Verification items for the finished model (mm, model axes). A direction names the side the tool comes from. Round coordinates to 2 decimals unless told otherwise and drop trailing zeros. Write each loop counter-clockwise with the first axis right and the second up, starting at its lowest first coordinate (ties: lowest second). Pieces come first, ordered by that corner, then holes.
from build123d import *

# Parameters (mm, degrees)
T_LE_DE_BASE_PLI_E1_DEPTH             = 20.5
ESQUISSE8_W                           = 24
ESQUISSE8_H                           = 2
BOSS_EXTRU_1_DEPTH                    = 8.5
T_LE_PLI_E_SUR_AR_TE1_STRIP_W         = 10
T_LE_PLI_E_SUR_AR_TE1_STRIP_H         = 2
T_LE_PLI_E_SUR_AR_TE1_STRIP_CUT_DEPTH = 8.5
T_LE_PLI_E_SUR_AR_TE1_DEPTH           = 8.5
ESQUISSE12_W                          = 1.5
ESQUISSE12_H                          = 12
ENL_V_MAT_EXTRU_1_DEPTH               = 8.5
DIAM_TRE_DU_PER_AGE_4_0_4_1_D         = 4
DIAM_TRE_DU_PER_AGE_8_0_8_1_D         = 8
DIAM_TRE_DU_PER_AGE_2_5_2_5_1_D       = 2.5
R_P_TITION_CIRCULAIRE1_COUNT          = 8
DIAM_TRE_DU_PER_AGE_4_0_4_2_D         = 4
DIAM_TRE_DU_PER_AGE_2_5_2_5_2_D       = 2.5
CONG_1_R                              = 4
DIAM_TRE_DU_PER_AGE_8_0_8_2_D         = 8
DIAM_TRE_DU_PER_AGE_2_5_2_5_3_D       = 2.5
R_P_TITION_CIRCULAIRE2_COUNT          = 4
CUT_EXTRUDE1_DEPTH                    = 54.200093985
CUT_EXTRUDE1_DEPTH_BACK               = 54.200093985
SKETCH1_R                             = 1.25


# Sheet-metal steps are written as plain solids
with BuildPart() as part:
    # Esquisse1 → Tôle de base pliée1 (new body)
    with BuildSketch(Plane(origin=(0, 0, 0), x_dir=(0, 0, -1), z_dir=(1, 0, 0))):
        with BuildLine():
            Line((0, 27), (0, 3))
            ThreePointArc((0, 3), (-0.878679656, 0.878679656), (-3, 0))
            Line((-3, 0), (-37.5, 0))
            Line((-37.5, 0), (-37.5, 2))
            Line((-37.5, 2), (-3, 2))
            ThreePointArc((-3, 2), (-2.292893219, 2.292893219), (-2, 3))
            Line((-2, 3), (-2, 27))
            Line((-2, 27), (0, 27))
        make_face()
    extrude(amount=T_LE_DE_BASE_PLI_E1_DEPTH)

    # Esquisse8 → Boss.-Extru.1 (add)
    with BuildSketch(Plane(origin=(20.5, 0, 0), x_dir=(0, 0, -1), z_dir=(1, 0, 0))):
        with Locations((-19, 1)):
            Rectangle(ESQUISSE8_W, ESQUISSE8_H)
    extrude(amount=BOSS_EXTRU_1_DEPTH)

    # Tôle pliée sur arête1 strip (across the edge) → Tôle pliée sur arête1 strip cut (cut)
    with BuildSketch(Plane(origin=(20.5, 2, 31), x_dir=(0, 0, -1), z_dir=(1, 0, 0))):
        with Locations((-4, -1)):
            Rectangle(T_LE_PLI_E_SUR_AR_TE1_STRIP_W, T_LE_PLI_E_SUR_AR_TE1_STRIP_H)
    extrude(amount=T_LE_PLI_E_SUR_AR_TE1_STRIP_CUT_DEPTH, mode=Mode.SUBTRACT)

    # Tôle pliée sur arête1 section (across the edge) → Tôle pliée sur arête1 (add)
    with BuildSketch(Plane(origin=(20.5, 2, 31), x_dir=(0, 0, -1), z_dir=(1, 0, 0))):
        with BuildLine():
            Line((-2, 1), (-2, 25))
            Line((-2, 25), (0, 25))
            Line((0, 25), (0, 1))
            ThreePointArc((0, 1), (0.292893219, 0.292893219), (1, 0))
            Line((1, 0), (1, -2))
            ThreePointArc((1, -2), (-1.121320344, -1.121320344), (-2, 1))
        make_face()
    extrude(amount=T_LE_PLI_E_SUR_AR_TE1_DEPTH)

    # Esquisse12 → Enlèv. mat.-Extru.1 (cut)
    with BuildSketch(Plane(origin=(0, 2, 0), x_dir=(1, 0, 0), z_dir=(0, 1, 0))):
        with Locations((19.75, -31.5)):
            Rectangle(ESQUISSE12_W, ESQUISSE12_H)
    extrude(amount=-ENL_V_MAT_EXTRU_1_DEPTH, mode=Mode.SUBTRACT)

    # Diamètre du perçage Ø4.0 (4)1 (through all)
    with Locations(Plane(origin=(0, 2, 0), x_dir=(1, 0, 0), z_dir=(0, 1, 0))):
        with Locations((24.25, -12.13), (24.25, -22.13)):
            Hole(DIAM_TRE_DU_PER_AGE_4_0_4_1_D / 2)

    # Diamètre du perçage Ø8.0 (8)1 (through all)
    with Locations(Plane(origin=(0, 2, 0), x_dir=(1, 0, 0), z_dir=(0, 1, 0))):
        with Locations((9.75, -25.5)):
            Hole(DIAM_TRE_DU_PER_AGE_8_0_8_1_D / 2)

    # Diamètre du perçage Ø2.5 (2.5)1 (through all)
    with Locations(Plane(origin=(0, 2, 0), x_dir=(1, 0, 0), z_dir=(0, 1, 0))):
        with Locations((9.75, -18.5)):
            diam_tre_du_per_age_2_5_2_5_1 = Hole(DIAM_TRE_DU_PER_AGE_2_5_2_5_1_D / 2)

    # Répétition circulaire1: Diamètre du perçage Ø2.5 (2.5)1 ×8 about axis, 3 skipped
    r_p_tition_circulaire1_axis = Axis((9.75, 2, 25.5), (0, 1, 0))
    add([diam_tre_du_per_age_2_5_2_5_1.rotate(r_p_tition_circulaire1_axis, i * 360 / R_P_TITION_CIRCULAIRE1_COUNT) for i in range(1, R_P_TITION_CIRCULAIRE1_COUNT) if i not in (1, 3, 6)], mode=Mode.SUBTRACT)

    # Diamètre du perçage Ø4.0 (4)2 (through all)
    with Locations(Plane.XY.offset(33)):
        with Locations((24.25, 19.87), (24.25, 9.87)):
            Hole(DIAM_TRE_DU_PER_AGE_4_0_4_2_D / 2)

    # Diamètre du perçage Ø2.5 (2.5)2 (through all)
    with Locations(Plane.XY.offset(2)):
        with Locations((10, 14.87)):
            Hole(DIAM_TRE_DU_PER_AGE_2_5_2_5_2_D / 2)

    # Congé1
    cong_1_edges = [part.edges().sort_by_distance(p)[0] for p in [
        (20.5, 27, 1),
        (29, 1, 7),
        (29, 27, 32),
        (19, 1, 37.5),
    ]]
    fillet(cong_1_edges, radius=CONG_1_R)

    # Symétrie1: part across plane


with BuildPart() as part_1:
    add(part.part)
    add(part.part.mirror(Plane(origin=(0, 3, 3), x_dir=(0, 0, 1), z_dir=(1, 0, 0))))

    # Diamètre du perçage Ø8.0 (8)2 (through all)
    with Locations(Plane(origin=(0, 2, 0), x_dir=(1, 0, 0), z_dir=(0, 1, 0))):
        with Locations((0, -12.13)):
            Hole(DIAM_TRE_DU_PER_AGE_8_0_8_2_D / 2)

    # Diamètre du perçage Ø2.5 (2.5)3 (through all)
    with Locations(Plane(origin=(0, 2, 0), x_dir=(1, 0, 0), z_dir=(0, 1, 0))):
        with Locations((0, -5.13)):
            diam_tre_du_per_age_2_5_2_5_3 = Hole(DIAM_TRE_DU_PER_AGE_2_5_2_5_3_D / 2)

    # Répétition circulaire2: Diamètre du perçage Ø2.5 (2.5)3 ×4 about axis
    r_p_tition_circulaire2_axis = Axis((0, 0, 12.13), (0, 1, 0))
    for i in range(1, R_P_TITION_CIRCULAIRE2_COUNT):
        add(diam_tre_du_per_age_2_5_2_5_3.rotate(r_p_tition_circulaire2_axis, i * 360 / R_P_TITION_CIRCULAIRE2_COUNT), mode=Mode.SUBTRACT)

    # Sketch1 → Cut-Extrude1 (cut, two sides: drawn at the far end of the back side and taken through both)
    with BuildSketch(Plane.XY.offset(2).offset(-CUT_EXTRUDE1_DEPTH_BACK)):
        with Locations((-10, 21.87)):
            Circle(SKETCH1_R)
        with Locations((-3, 14.87)):
            Circle(SKETCH1_R)
        with Locations((-10, 7.87)):
            Circle(SKETCH1_R)
        with Locations((-17, 14.87)):
            Circle(SKETCH1_R)
        with Locations(Location((3, 14.87, 0), (0, 0, 90))):
            Circle(SKETCH1_R)
        with Locations(Location((10, 7.87, 0), (0, 0, 90))):
            Circle(SKETCH1_R)
        with Locations(Location((17, 14.87, 0), (0, 0, 90))):
            Circle(SKETCH1_R)
        with Locations(Location((10, 21.87, 0), (0, 0, 90))):
            Circle(SKETCH1_R)
    extrude(amount=CUT_EXTRUDE1_DEPTH + CUT_EXTRUDE1_DEPTH_BACK, mode=Mode.SUBTRACT)


solid = part_1.part
Q1. Depth check by flat-ended pin: P1, Ø2, axis at x = 2.75, z = 25.5, coming from the +Y side; P2, Ø4, axis at y = 14, z = 30.5, coming from the -X side; P3, Ø12, axis at x = -7.5, z = 30.5, coming from the +Y side; P4, Ø8, axis at y = 11, z = 5.5, coming from the -X side. Enter the tip coordinate at first touch or a pass-through.
Recorded:
P1: passes through
P2: stops at x = -29
P3: stops at y = 2
P4: stops at x = -20.5
Q2. Material ranges on line 1 along Z through (x, y) = (-9.75, 1); line 2 along Y through (x, z) = (-24.25, 32.5); line 3 along X through (y, z) = (0.8, 5.13), recorded low to high.
Recorded:
line 1: z = 0.76 to 17.25, 19.75 to 21.5, 29.5 to 31.25, 33.75 to 37.5
line 2: y = 1.34 to 7.87, 11.87 to 17.87, 21.87 to 27
line 3: x = -20.5 to -1.25, 1.25 to 20.5
Q3. Sectioned sample at A-A (y = 5.75). Enter the section's corners in (x, z).
Recorded:
outline: (-29, 31) - (-20.5, 31) - (-20.5, 33) - (-29, 33) - close; (-20.5, 0) - (20.5, 0) - (20.5, 2) - (-20.5, 2) - close; (20.5, 31) - (29, 31) - (29, 33) - (20.5, 33) - close
Q4. Sectioned sample at B-B (x = -24.25). Enter the section's corners in (y, z), plus the area to 3 significant figures.
Recorded:
outline: (0, 7) - (2, 7) - (2, 10.13) - (0, 10.13) - close; (0, 14.13) - (2, 14.13) - (2, 20.13) - (0, 20.13) - close; (0, 24.13) - (2, 24.13) - (2, 30) arc R1 cw to (3, 31) - (7.87, 31) - (7.87, 33) - (3, 33) arc R3 ccw to (0, 30) - close; (11.87, 31) - (17.87, 31) - (17.87, 33) - (11.87, 33) - close; (21.87, 31) - (27, 31) - (27, 33) - (21.87, 33) - close
area: 68.3 mm2
Q5. Tool access check on faces 5 (the flat face through (-20.5, 12, 32)), 6 (the flat face through (0, 0, 24)), 7 (the cylindrical face through (24.69, 0.86, 32.1)), 8 (the cylindrical face through (-8.5, 0.99, 32.55)), 9 (the flat face through (-23, 1, 7)). Record the directions out of +Z, -Z, +X, -X, +Y, -Y that give a thin tool (end or side, any length) a straight path to the whole face; none if there is none.
Recorded:
face 5: +Z, +Y, -Y
face 6: +Z, -Z, +X, -X, -Y
face 7: +Z, +X, -Y
face 8: +Y, -Y
face 9: -Z, -X, +Y, -Y
Q6. Release check for a two-part mould opening along Z. For faces 1 (the flat face through (20, 1, 25.5)), 2 (the cylindrical face through (-26.248, 0.986, 12.042)), 3 (the cylindrical face through (-15.81, 15.25, 0.99)), 4 (the cylindrical face through (-10.271, 0.986, 21.534)) record: released by +Z, released by -Z, zero draft, split by the parting line, or undercut.
Recorded:
face 1: released by +Z
face 2: undercut
face 3: zero draft
face 4: undercut
Q7. Sectioned sample at C-C (x = 0). Enter the section's corners in (y, z).
Recorded:
outline: (0, 3) arc R3 ccw to (3, 0) - (27, 0) - (27, 2) - (3, 2) arc R1 cw to (2, 3) - (2, 3.88) - (0, 3.88) - close; (0, 6.38) - (2, 6.38) - (2, 8.13) - (0, 8.13) - close; (0, 16.13) - (2, 16.13) - (2, 17.88) - (0, 17.88) - close; (0, 20.38) - (2, 20.38) - (2, 37.5) - (0, 37.5) - close
Q8. Sectioned sample at D-D (z = 18.5). Enter the section's corners in (x, y), plus the area to 3 significant figures.
Recorded:
outline: (-29, 0) - (-11, 0) - (-11, 2) - (-29, 2) - close; (-8.5, 0) - (-1.08, 0) - (-1.08, 2) - (-8.5, 2) - close; (1.08, 0) - (8.5, 0) - (8.5, 2) - (1.08, 2) - close; (11, 0) - (29, 0) - (29, 2) - (11, 2) - close
area: 102 mm2
